from build123d import *

# Parameters (mm, degrees)
F0_W     = 22
F0_H     = 6
F0_R     = 1.325
F1_DEPTH = 16
F2_R     = 16
F3_DEPTH = 5


with BuildPart() as f1:
    # F0 (on Top) → F1 (new body)
    with BuildSketch(Plane.XY):
        Rectangle(F0_W, F0_H)
        with Locations((-8, 0)):
            Circle(F0_R, mode=Mode.SUBTRACT)
    extrude(amount=F1_DEPTH)

    # F2 (on Front) → F3 (cut, symmetric)
    with BuildSketch(Plane.XZ):
        with Locations((11, 16)):
            Circle(F2_R)
    extrude(amount=F3_DEPTH, both=True, mode=Mode.SUBTRACT)


solid = f1.part
Source: CAD feature listing. Evaluate the final solid. Frame: model axes, mm. Coordinates: 2 decimals unless noted, no trailing zeros. Order: outer loops, then holes, each group sorted by start corner. A loop starts at its lowest first (then second) coordinate and runs counter-clockwise, first axis right, second up.
Item 1: Cut plane B-B (y = 0). Return loops of the section in (x, z) (3 decimals), plus the area to 3 significant figures.
Output values:
outline: (-11, 0) - (-9.325, 0) - (-9.325, 16) - (-11, 16) - close; (-6.675, 0) - (11, 0) arc R16 cw to (-5, 16) - (-6.675, 16) - close
area: 109 mm2
Item 2: Material intervals for line 1 (Y direction, x = -8, z = 4) (3 decimals); line 2 (X direction, y = -0.25, z = 15.5); line 3 (X direction, y = -1.2, z = 6.5), sorted ascending.
Output values:
line 1: y = -3 to -1.325, 1.325 to 3
line 2: x = -11 to -9.3, -6.7 to -4.99
line 3: x = -11 to -8.56, -7.44 to -1.87
Item 3: Cut plane A-A (x = -8). Return loops of the section in (y, z) (3 decimals), plus the area to 3 significant figures.
Output values:
outline: (-3, 0) - (-1.325, 0) - (-1.325, 16) - (-3, 16) - close; (1.325, 0) - (3, 0) - (3, 16) - (1.325, 16) - close
area: 53.6 mm2
Item 4: Pull-direction query (X, two-part tool) for faces 1 (the face through (-11, 0, 8)), 2 (the face through (-6.736, 0.398, 7.888)), 3 (the face through (0, 0, 0)); classes: pulls with the +X half, pulls with the -X half, needs draft (parallel to the pull), parting line crosses it, or undercut.
Output values:
face 1: pulls with the -X half
face 2: undercut
face 3: needs draft
Item 5: First-contact query: P1, Ø2, axis at x = -0.5, y = 1.5, coming from the +Z side. Flat tip, straight axial feed; report the tip coordinate or a pass-through.
Output values:
P1: stops at z = 6.01
Item 6: Cut plane C-C (z = 14.5). Return loops of the section in (x, y) (3 decimals), plus the area to 3 significant figures.
Output values:
outline: (-11, -3) - (-4.93, -3) - (-4.93, 3) - (-11, 3) - close; hole circle Ø2.65 at (-8, 0)
area: 30.9 mm2
Item 7: Cut plane D-D (y = -2). Return loops of the section in (x, z), plus the area to 3 significant figures.
Output values:
outline: (-11, 0) - (11, 0) arc R16 cw to (-5, 16) - (-11, 16) - close
area: 151 mm2
